from build123d import *

# Parameters (mm, degrees)
F1_DEPTH = 25.4
F2_R     = 5.08


with BuildPart() as f1:
    # F0 (on Front) → F1 (new body)
    with BuildSketch(Plane.XZ):
        Polygon((-11.43, 14.737148), (-11.43, 17.277148), (0, 18.277143), (11.43, 17.277148), (11.43, 14.737148), (8.255, 14.737148), (8.255, 13.721148), (15.24, 13.721148), (15.24, 19.940279), (0, 20.697519), (-15.24, 19.940279), (-15.24, 13.721148), (-8.255, 13.721148), (-8.255, 14.737148), align=None)
    extrude(amount=F1_DEPTH)

    # F2
    f2_edges = [f1.edges().sort_by_distance(p)[0] for p in [
        (15.24, -12.7, 19.940279),
        (-15.24, -12.7, 19.940279),
    ]]
    fillet(f2_edges, radius=F2_R)


solid = f1.part
Verification items for the finished model (mm, model axes). A direction names the side the tool comes from. Coordinates: 2 decimals unless noted, no trailing zeros. Order: outer loops, then holes, each group sorted by start corner. A loop starts at its lowest first (then second) coordinate and runs counter-clockwise, first axis right, second up. Notation, with made-up numbers: M 76.5,31.5 L 89.5,31.5 A32 cw 89.5,65.5 Z; hole C 52.25,59.25 d8. An arc over 180 degrees is marked long. Return JSON: item names as keys, results as strings.
1) Cross-section at A-A, the plane z = 16.5. Record the boundary of the cut face in (x, y).
Answer list:
{"outline": "M -15.05,-25.4 L -11.43,-25.4 L -11.43,0 L -15.05,0 Z; M 11.43,-25.4 L 15.05,-25.4 L 15.05,0 L 11.43,0 Z"}
2) Cross-section at D-D, the plane x = 13. Record the boundary of the cut face in (y, z), and give its area (3 significant figures).
Answer list:
{"outline": "M -25.4,13.72 L 0,13.72 L 0,19.32 L -25.4,19.32 Z", "area": "142 mm2"}
3) Release check for a two-part mould opening along Z. For faces 1 (the flat face through (-8.255, -13, 14)), 2 (the cylindrical face through (-13.8, -12.88, 18.65)), 3 (the flat face through (10, -13, 14.737)), 4 (the flat face through (12, -13, 13.721)) record: +Z half, -Z half, draft (parallel to the pull), parting line (faces both ways), or undercut.
Answer list:
{"face 1": "draft", "face 2": "+Z half", "face 3": "undercut", "face 4": "-Z half"}
4) Thickness scan on L1, parallel to X at y = -22.25, z = 15.25; L2, parallel to X at y = -11.75, z = 17; L3, parallel to Z at x = 7.5, y = -12.5. Record the ranges inside material, lowest first. Write a range as [from, to].
Answer list:
{"L1": "[-15.24, -11.43], [11.43, 15.24]", "L2": "[-14.87, -11.43], [11.43, 14.87]", "L3": "[17.62, 20.32]"}
5) Access from +Z, -Z, +X, -X, +Y, -Y to the whole of each face (thin tool, end or side, straight path). Record for faces 5 (the flat face through (-5.8, -12.52, 17.77)), 6 (the flat face through (-15.24, -13, 14)), 7 (the flat face through (8.255, -13, 14)).
Answer list:
{"face 5": "+Y, -Y", "face 6": "+Z, -Z, -X, +Y, -Y", "face 7": "-Z, +Y, -Y"}
6) Gauge pin test, flat ends, axial feed: pin 1 (1.6 mm diameter, centred on x = -9.5, y = -8.5, fed in from +Z); pin 2 (5 mm diameter, centred on x = -3, y = -15.5, fed in from +Z); pin 3 (1.5 mm diameter, centred on x = 4.5, y = -19.5, fed in from -Z); pin 4 (2 mm diameter, centred on x = -0.5, z = 16.5, fed in from +Y). Record the tip position at first contact, or that the pin passes through.
Answer list:
{"pin 1": "z = 20.27", "pin 2": "z = 20.67", "pin 3": "z = 17.82", "pin 4": "through"}
7) Cross-section at C-C, the plane x = -9.5. Record the boundary of the cut face in (y, z), and give its area (3 significant figures).
Answer list:
{"outline": "M -25.4,13.72 L 0,13.72 L 0,14.74 L -25.4,14.74 Z; M -25.4,17.45 L 0,17.45 L 0,20.23 L -25.4,20.23 Z", "area": "96.4 mm2"}
8) Cross-section at B-B, the plane y = -15.25. Record the boundary of the cut face in (x, z) (3 decimals).
Answer list:
{"outline": "M -15.24,13.721 L -8.255,13.721 L -8.255,14.737 L -11.43,14.737 L -11.43,17.277 L 0,18.277 L 11.43,17.277 L 11.43,14.737 L 8.255,14.737 L 8.255,13.721 L 15.24,13.721 L 15.24,15.106 A5.08 ccw 10.412,20.18 L 0,20.698 L -10.412,20.18 A5.08 ccw -15.24,15.106 Z"}
